Here's how the part is built. I have some questions about the finished solid (model axes, mm). A direction names the side the tool comes from. Give positions to 0.01 mm unless a question says otherwise; leave off trailing zeros. Loops run counter-clockwise (first coordinate to the right, second up) from the corner with the lowest first, then second, coordinate; pieces in that order, holes last.
Q1. For faces 1 (the face through (2, 3, 0)), 2 (the face through (0, 0, 0)), which set-ups out of +Z, -Z, +X, -X, +Y, -Y let a thin tool reach every point of the face, with its end or its side?
Q2. I'm going to push flat-ended pins straight in: P1, Ø2, axis at y = 4, z = -1.5, coming from the -X side; P2, Ø0.6, axis at y = 4, z = 2.5, coming from the +X side; P3, Ø1.5, axis at x = -0.5, z = -0.5, coming from the +Y side. Where does each tip first touch, or does it pass through?
Q3. Suppose I cut it at B-B (z = 0). List the corners of the cut face in (x, y) for me, and give its area (3 significant figures).
Q4. Suppose I cut it at C-C (y = 2.4). List the corners of the cut face in (x, z) for me.
Q5. Suppose I cut it at D-D (z = 1.55). List the corners of the cut face in (x, y) for me, and give its area (3 significant figures).
Q6. I need wall thicknesses on probe 1 along Z at (x, y) = (-0.55, 0.9); probe 2 along Y at (x, z) = (-1.6, -0.8). Which ranges of each line are inside material? Lowest first, please.
Q7. Thinking about a two-plate mould opening in Z: for faces 3 (the face through (2.5, 2, 0)), 4 (the face through (0, 0.5, 0)), 5 (the face through (-1.15, 1.91, -2.5)), 6 (the face through (1.15, 1.91, 2.5)), which applies, pulls with the +Z half, pulls with the -Z half, needs draft (parallel to the pull), parting line crosses it, or undercut?
Q8. Suppose I cut it at A-A (x = 0). List the corners of the cut face in (y, z) for me.
Autodesk Inventor part; units mm, degrees
ref_plane "YZ Plane" through (0, 0, 0) normal (1, 0, 0) x (0, 1, 0)
ref_plane "XZ Plane" through (0, 0, 0) normal (0, 1, 0) x (-1, 0, 0)
ref_plane "XY Plane" through (0, 0, 0) normal (0, 0, 1) x (1, 0, 0)
sketch "Sketch1" plane through (0, 0, 0) normal (0, 1, 0) x (-1, 0, 0)
  line L0 (-2.5, 2.5) -> (2.5, 2.5)
  line L1 (2.5, 2.5) -> (2.5, -2.5)
  line L2 (2.5, -2.5) -> (-2.5, -2.5)
  line L3 (-2.5, -2.5) -> (-2.5, 2.5)
  line L4 (-2.5, 2.5) -> (2.5, -2.5) construction
  line L5 (2.5, 2.5) -> (-2.5, -2.5) construction
  point P0 (0, 0)
  dimension "d0" = 5
  dimension "d1" = 5
extrude "Extrusion1" add sketch "Sketch1" along normal blind 5
shell "Shell1" thickness 0.5 removed faces 1 at (-0.8333, 5, -0.8333)
sketch "Sketch3" plane through (-2.5, 0, 2.5) normal (0, 0, 1) x (1, 0, 0)
  line L0 (2.5, 9.1674) -> (2.5, 2.1156) construction
  line L1 (1.4995, 9.1674) -> (1.4995, 2.1156)
  line L2 (3.5005, 2.1156) -> (3.5005, 9.1674)
  arc A0 (3.5005, 9.1674) -> (1.4995, 9.1674) centre (2.5, 9.1674) ccw
  arc A1 (1.4995, 2.1156) -> (3.5005, 2.1156) centre (2.5, 2.1156) ccw
  point P0 (2.5, 0)
  point P1 (2.5, 5.6415)
extrude "Extrusion3" cut sketch "Sketch3" against normal through all
sketch "Sketch4" plane through (0, 5, 0) normal (0, 1, 0) x (1, 0, 0)
  point P0 (0, 0)
sketch "Sketch5" plane through (0, 5, 0) normal (0, 1, 0) x (1, 0, 0)
  point P0 (0, 0)
sketch "Sketch6" plane through (0, 5, 0) normal (0, 1, 0) x (1, 0, 0)
  point P0 (0, 0)
sketch "Sketch7" plane through (0, 0, 0) normal (0, -1, 0) x (1, 0, 0)
  point P0 (0, 0)
sketch "Sketch8" plane through (-2.5, 0, -2.5) normal (-1, 0, 0) x (0, 0, 1)
  point P0 (2.5, 0)
sketch "Sketch9" plane through (2.5, 0, 2.5) normal (1, 0, 0) x (0, 0, -1)
  line L0 (1.5, 3.5) -> (3.5, 3.5)
  line L1 (3.5, 3.5) -> (3.5, 4.5)
  line L2 (3.5, 4.5) -> (1.5, 4.5)
  line L3 (1.5, 4.5) -> (1.5, 3.5)
  line L4 (1.5, 3.5) -> (3.5, 4.5) construction
  line L5 (3.5, 3.5) -> (1.5, 4.5) construction
  line L6 (0, 5) -> (5, 5)
  point P0 (2.5, 0)
  point P1 (2.5, 4)
  dimension "d10" = 1
  dimension "d14" = 2
  dimension "d15" = 1
extrude "Extrusion4" add sketch "Sketch9" along normal blind 0.4 draft -30
sketch "Sketch10" plane through (-2.5, 0, -2.5) normal (-1, 0, 0) x (0, 0, 1)
  line L0 (1.5, 3.5) -> (3.5, 3.5)
  line L1 (3.5, 3.5) -> (3.5, 4.5)
  line L2 (3.5, 4.5) -> (1.5, 4.5)
  line L3 (1.5, 4.5) -> (1.5, 3.5)
  line L4 (1.5, 3.5) -> (3.5, 4.5) construction
  line L5 (3.5, 3.5) -> (1.5, 4.5) construction
  line L6 (0, 5) -> (5, 5)
  point P0 (2.5, 0)
  point P1 (2.5, 4)
  dimension "d13" = 1
  dimension "d16" = 2
  dimension "d17" = 1
extrude "Extrusion5" add sketch "Sketch10" along normal blind 0.4 draft -30
equation "\"d16\" = d14"
equation "\"d17\" = d15"
properties part number "snapfit_v09"
Solutions:
1. face 1: +Y
1. face 2: +Z, -Z, +X, -X, -Y
2. P1: stops at x = -2.9
2. P2: stops at x = 2.5
2. P3: stops at y = 0.5
3. outline: (-2.9, 3.73) - (-2.5, 3.5) - (-2.5, 0) - (2.5, 0) - (2.5, 3.5) - (2.9, 3.73) - (2.9, 4.27) - (2.5, 4.5) - (2.5, 5) - (2, 5) - (2, 0.5) - (-2, 0.5) - (-2, 5) - (-2.5, 5) - (-2.5, 4.5) - (-2.9, 4.27) - close
3. area: 7.62 mm2
4. outline: (-2.5, -2.5) - (-1, -2.5) - (-1, -2) - (-2, -2) - (-2, 2) - (-1, 2) - (-1, 2.5) - (-2.5, 2.5) - close; (1, -2.5) - (2.5, -2.5) - (2.5, 2.5) - (1, 2.5) - (1, 2) - (2, 2) - (2, -2) - (1, -2) - close
5. outline: (-2.5, 0) - (2.5, 0) - (2.5, 5) - (2, 5) - (2, 0.5) - (-2, 0.5) - (-2, 5) - (-2.5, 5) - close
5. area: 7.00 mm2
6. probe 1: z = -2.5 to -2, 2 to 2.5
6. probe 2: y = 0 to 0.5
7. face 3: needs draft
7. face 4: undercut
7. face 5: pulls with the -Z half
7. face 6: pulls with the +Z half
8. outline: (0, -2.5) - (1.12, -2.5) - (1.12, -2) - (0.5, -2) - (0.5, 2) - (1.12, 2) - (1.12, 2.5) - (0, 2.5) - close
